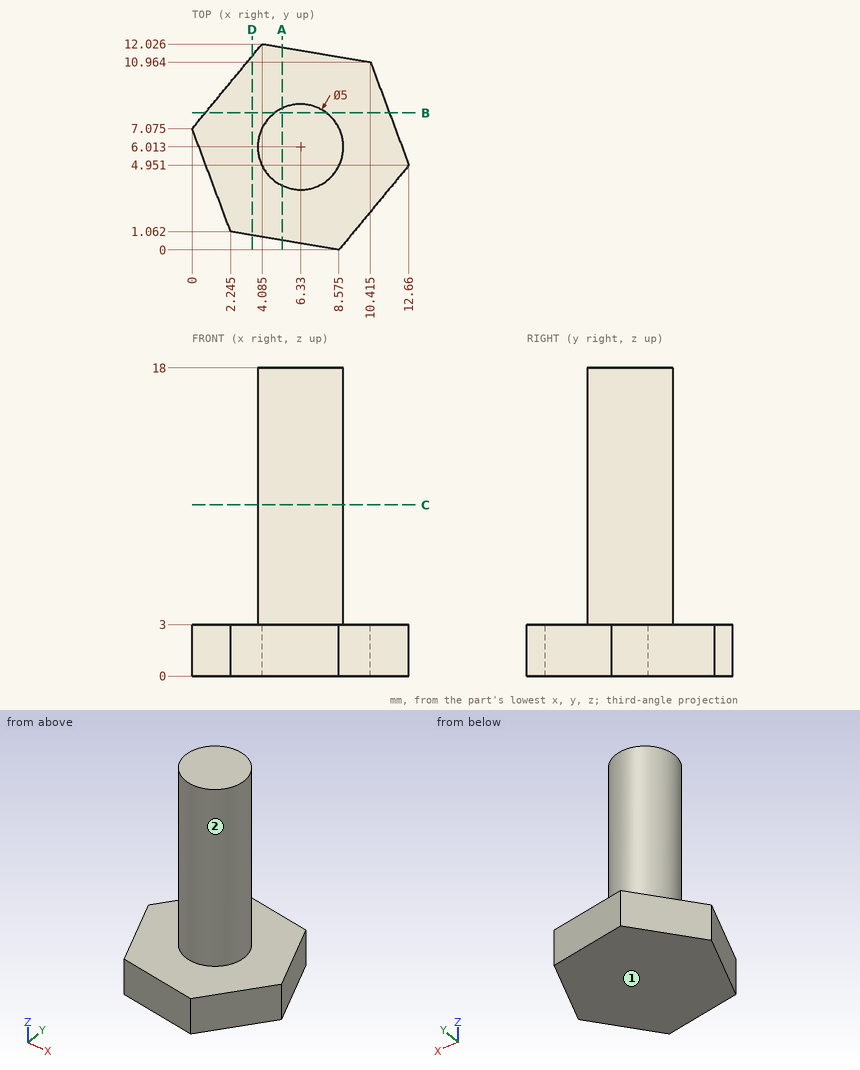
Input: dimensioned drawing with shaded views. Units: mm. Origin: part minimum x, y, z. A direction names the side the tool comes from. Round coordinates to 2 decimals unless told otherwise and drop trailing zeros. Order: outer loops, then holes, each group sorted by start corner. A loop starts at its lowest first (then second) coordinate and runs counter-clockwise, first axis right, second up.
Q1. Access query for the marked faces 1 and 2. Directions: +Z, -Z, +X, -X, +Y, -Y. A direction counts if a zero-diameter tool reaches every point of the face in a straight line with its end or side. Return the directions, or none.
Result sheet:
face 1: -Z, +X, -X, +Y, -Y
face 2: +Z
Q2. Pin query (flat end, axial travel): pin 1 (1 mm diameter, centred on y = 11, z = 8.5, fed in from +X); pin 2 (5 mm diameter, centred on y = 5.5, z = 12.5, fed in from -X); pin 3 (1.5 mm diameter, centred on x = 6.5, z = 2.5, fed in from -Y); pin 4 (6 mm diameter, centred on y = 2, z = 8.5, fed in from -X). Return the tip coordinate at first contact, or that it passes through.
Result sheet:
pin 1: passes through
pin 2: stops at x = 3.83
pin 3: stops at y = 0.22
pin 4: stops at x = 4.04
Q3. Material intervals for probe 1 along Z at (x, y) = (11, 3.5); probe 2 along Y at (x, z) = (6.5, 10.5); probe 3 along Y at (x, z) = (5.75, 4.25) (1 decimal), sorted ascending.
Result sheet:
probe 1: z = 0 to 3
probe 2: y = 3.52 to 8.51
probe 3: y = 3.6 to 8.4
Q4. Section D-D, the plane x = 3.5. Output: boundary loops of the cut face in (y, z), and give its area (3 significant figures).
Result sheet:
outline: (0.85, 0) - (11.32, 0) - (11.32, 3) - (0.85, 3) - close
area: 31.4 mm2
Q5. Section A-A, the plane x = 5.25. Output: boundary loops of the cut face in (y, z).
Result sheet:
outline: (0.56, 0) - (11.83, 0) - (11.83, 3) - (8.27, 3) - (8.27, 18) - (3.76, 18) - (3.76, 3) - (0.56, 3) - close
Q6. Section B-B, the plane y = 8. Output: boundary loops of the cut face in (x, z).
Result sheet:
outline: (0.76, 0) - (11.52, 0) - (11.52, 3) - (7.85, 3) - (7.85, 18) - (4.81, 18) - (4.81, 3) - (0.76, 3) - close
Q7. Section C-C, the plane z = 10. Output: boundary loops of the cut face in (x, y), and give its area (3 significant figures).
Result sheet:
outline: circle Ø5 at (6.33, 6.01)
area: 19.6 mm2
